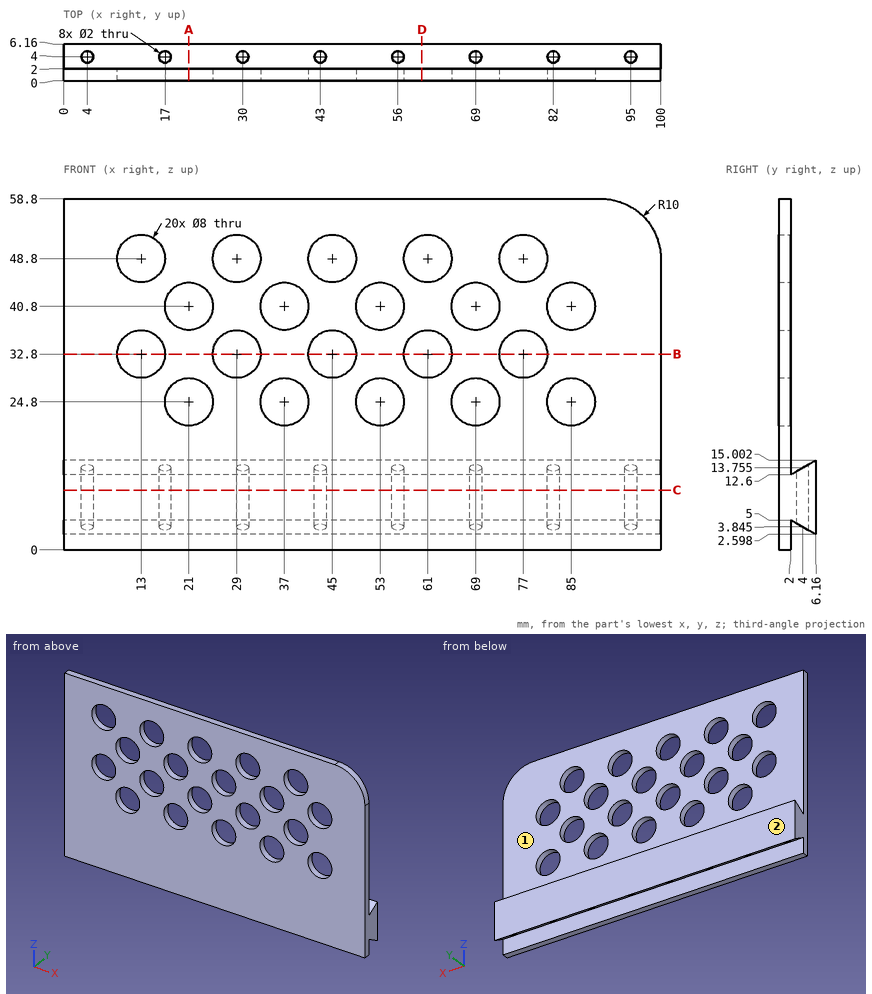
Could you check a few things on this drawing? It's one solid part, dimensions in mm from its lowest x, y, z. A direction names the side the tool comes from. Round coordinates to 2 decimals unless told otherwise and drop trailing zeros. Write each loop counter-clockwise with the first axis right and the second up, starting at its lowest first coordinate (ties: lowest second). Pieces come first, ordered by that corner, then holes. Notation, with made-up numbers: (69, -4) -> (76, -4) arc R22 cw to (76, 4) -> close; hole circle Ø8 at (85, 50.25). An arc over 180 degrees is marked (long way). One line per item, written item: value.
1) Suppose I cut it at C-C on z = 10. Give the number of separate pieces and of enclosed holes in the cut face, plus the area to 3 significant figures.
Filled sheet:
separate pieces: 1
enclosed holes: 8
area: 591 mm2
2) I'm going to push flat-ended pins straight in: pin 1 Ø13 at (x, z) = (29, 48.8) entering from +Y; pin 2 Ø1 at (x, y) = (51.5, 4.5) entering from +Z; pin 3 Ø2 at (x, y) = (69.5, 5) entering from +Z. Where does each tip first touch, or does it pass through?
Filled sheet:
pin 1: stops at y = 2
pin 2: stops at z = 14.33
pin 3: stops at z = 14.91
3) Suppose I cut it at B-B on z = 32.8. List the corners of the cut face in (x, y) for me, plus the area to 3 significant figures.
Filled sheet:
outline: (0, 0) -> (9, 0) -> (9, 2) -> (0, 2) -> close; (17, 0) -> (25, 0) -> (25, 2) -> (17, 2) -> close; (33, 0) -> (41, 0) -> (41, 2) -> (33, 2) -> close; (49, 0) -> (57, 0) -> (57, 2) -> (49, 2) -> close; (65, 0) -> (73, 0) -> (73, 2) -> (65, 2) -> close; (81, 0) -> (100, 0) -> (100, 2) -> (81, 2) -> close
area: 120 mm2
4) Suppose I cut it at D-D on x = 60. List the corners of the cut face in (y, z) for me.
Filled sheet:
outline: (0, 0) -> (2, 0) -> (2, 5) -> (6.16, 2.6) -> (6.16, 15) -> (2, 12.6) -> (2, 28.93) -> (0, 28.93) -> close; (0, 36.67) -> (2, 36.67) -> (2, 44.93) -> (0, 44.93) -> close; (0, 52.67) -> (2, 52.67) -> (2, 58.8) -> (0, 58.8) -> close
5) If I drill on line 1 (X direction, y = 0.9, z = 48.8); line 2 (Z direction, x = 13, y = 0.95); line 3 (Z direction, x = 69, y = 1.3), over which ranges is the centre line in solid material (lowest first)? Write a range as [from, to].
Filled sheet:
line 1: x = [0, 9], [17, 25], [33, 41], [49, 57], [65, 73], [81, 100]
line 2: z = [0, 28.8], [36.8, 44.8], [52.8, 58.8]
line 3: z = [0, 20.8], [28.8, 36.8], [44.8, 58.8]
6) Suppose I cut it at A-A on x = 21. List the corners of the cut face in (y, z) for me, plus the area to 3 significant figures.
Filled sheet:
outline: (0, 0) -> (2, 0) -> (2, 5) -> (6.16, 2.6) -> (6.16, 15) -> (2, 12.6) -> (2, 20.8) -> (0, 20.8) -> close; (0, 28.8) -> (2, 28.8) -> (2, 36.8) -> (0, 36.8) -> close; (0, 44.8) -> (2, 44.8) -> (2, 58.8) -> (0, 58.8) -> close
area: 127 mm2
7) For the marked faces 1 and 2, which set-ups out of +Z, -Z, +X, -X, +Y, -Y let a thin tool reach every point of the face, with its end or its side?
Filled sheet:
face 1: +Z, +X, -X
face 2: +Z, -Z, +X, -X, +Y
